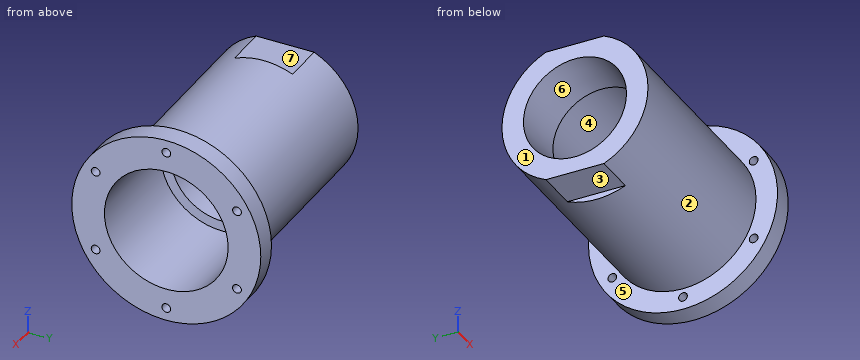
```python
from build123d import *

# Parameters (mm, degrees)
F0_R      = 42.5
F1_DEPTH  = 66.5
F2_R      = 55
F3_DEPTH  = 12
F5_D      = 5.1054
F6_R      = 30
F7_DEPTH  = 30
F7_TAPER  = 3
F8_R      = 30
F9_DEPTH  = 103
F11_R     = 36
F12_DEPTH = 63
F13_W     = 105.4392717779
F13_H     = 18.3104768991
F14_DEPTH = 24


with BuildPart() as f1:
    # F0 (on Right) → F1 (new body, symmetric)
    with BuildSketch(Plane.YZ):
        Circle(F0_R)
    extrude(amount=F1_DEPTH, both=True)

    # F2 (on face) → F3 (join)
    with BuildSketch(Plane.YZ.offset(66.5)):
        Circle(F2_R)
    extrude(amount=-F3_DEPTH)

    # F5 (through all)
    with Locations(Plane.YZ.offset(66.5)):
        with Locations((0, 47.5), (-41.1362066798, 23.75), (-41.1362066798, -23.75), (0, -47.5), (41.1362066798, -23.75), (41.1362066798, 23.75)):
            Hole(F5_D / 2)

    # F6 (on face) → F7 (cut)
    with BuildSketch(Plane(origin=(-66.5, 0, 0), x_dir=(0, -1, 0), z_dir=(-1, 0, 0))):
        Circle(F6_R)
    extrude(amount=-F7_DEPTH, taper=F7_TAPER, mode=Mode.SUBTRACT)

    # F8 (on face) → F9 (cut, through all)
    with BuildSketch(Plane.YZ.offset(66.5)):
        Circle(F8_R)
    extrude(amount=-F9_DEPTH, mode=Mode.SUBTRACT)

    # F11 (on offset) → F12 (cut, through all)
    with BuildSketch(Plane.YZ.offset(3.5)):
        Circle(F11_R)
    extrude(amount=F12_DEPTH, mode=Mode.SUBTRACT)

    # F13 (on face) → F14 (cut)
    with BuildSketch(Plane(origin=(-66.5, 0, 0), x_dir=(0, -1, 0), z_dir=(-1, 0, 0))):
        with Locations((-0.2345982939, 48.1552384496)):
            Rectangle(F13_W, F13_H)
        with Locations((-0.2345982939, -48.1552384496)):
            Rectangle(F13_W, F13_H)
    extrude(amount=-F14_DEPTH, mode=Mode.SUBTRACT)


solid = f1.part
```
Check sheet for the modelled part. Datum: model origin and axes. Units: mm. Face numbers are marked on the shaded views. A direction names the side the tool comes from. Coordinates: 2 decimals unless noted, no trailing zeros. Write each loop counter-clockwise with the first axis right and the second up, starting at its lowest first coordinate (ties: lowest second). Pieces come first, ordered by that corner, then holes. Notation, with made-up numbers: (47, 31.25) -> (93, 31.25) arc R20 cw to (93, 37.25) -> close; hole circle Ø3 at (-1.5, -37.5). An arc over 180 degrees is marked (long way). Use a Markdown table: item, result.
1. Tool access check on the marked faces 1, 2, 3 and 4. Record the directions out of +Z, -Z, +X, -X, +Y, -Y that give a thin tool (end or side, any length) a straight path to the whole face; none if there is none.
Reported:
| item | result |
|---|---|
| face 1 | +Z, -Z, -X, +Y, -Y |
| face 2 | -X |
| face 3 | -Z, -X, +Y, -Y |
| face 4 | +X |
2. Sectioned sample at A-A (x = -3). Enter the section's corners in (y, z), plus the area to 3 significant figures.
Reported:
| item | result |
|---|---|
| outline | circle Ø85 at (0, 0); hole circle Ø60 at (0, 0) |
| area | 2,850 mm2 |
3. Go/stop test with flat-tipped pins: pin 1 Ø3 at (x, z) = (28.5, -5.5) entering from -Y; pin 2 Ø12 at (x, y) = (-51, -2) entering from +Z; pin 3 Ø10 at (x, y) = (-22.5, 2) entering from +Z. Record where each tip stops, or that it passes through.
Reported:
| item | result |
|---|---|
| pin 1 | stops at y = -42.31 |
| pin 2 | stops at z = 39 |
| pin 3 | stops at z = 42.5 |
4. Scan lines: line 1 along Z through (x, y) = (58.25, 0); line 2 along X through (y, z) = (-30, 34); line 3 along Y through (x, z) = (7, -17). Record each from-to range of solid material in increasing order.
Reported:
| item | result |
|---|---|
| line 1 | z = -55 to -50.05, -44.95 to -36, 36 to 44.95, 50.05 to 55 |
| line 2 | x = 54.5 to 66.5 |
| line 3 | y = -38.95 to -31.73, 31.73 to 38.95 |
5. Sectioned sample at C-C (z = -47.5). Enter the section's corners in (x, y), plus the area to 3 significant figures.
Reported:
| item | result |
|---|---|
| outline | (54.5, -27.73) -> (66.5, -27.73) -> (66.5, -2.55) -> (54.5, -2.55) -> close; (54.5, 2.55) -> (66.5, 2.55) -> (66.5, 27.73) -> (54.5, 27.73) -> close |
| area | 604 mm2 |
6. Release check for a two-part mould opening along Z. For the marked faces 5, 6 and 7 record: pulls with the +Z half, pulls with the -Z half, needs draft (parallel to the pull), parting line crosses it, or undercut.
Reported:
| item | result |
|---|---|
| face 5 | needs draft |
| face 6 | undercut |
| face 7 | pulls with the +Z half |
7. Sectioned sample at B-B (y = 0). Give the number of separate pieces and of enclosed holes in the cut face, plus the area to 3 significant figures.
Reported:
| item | result |
|---|---|
| separate pieces | 4 |
| enclosed holes | 0 |
| area | 2,630 mm2 |
